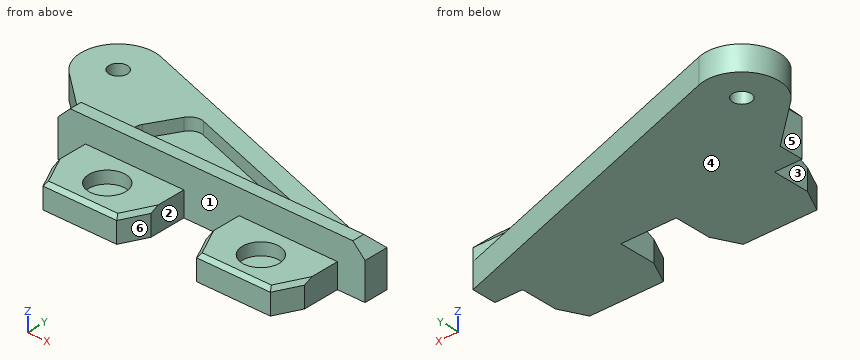
from build123d import *

# Parameters (mm, degrees)
SKIZZE1_R                       = 0.75
AUFSATZ_LINEAR_AUSTRAGEN1_DEPTH = 2
SKIZZE2_R                       = 1.5
SCHNITT_LINEAR_AUSTRAGEN1_DEPTH = 1
SKIZZE3_W                       = 25
SKIZZE3_H                       = 2
AUFSATZ_LINEAR_AUSTRAGEN2_DEPTH = 2
FASE1_SIZE                      = 1
SCHNITT_LINEAR_AUSTRAGEN2_DEPTH = 1
VERRUNDUNG1_R                   = 1
VERRUNDUNG2_R                   = 0.5
FASE2_SIZE                      = 0.3


with BuildPart() as part:
    # Skizze1 → Aufsatz-Linear austragen1 (new body)
    with BuildSketch(Plane.XY):
        with BuildLine():
            Line((9.25, -5), (3.25, -5))
            Line((3.25, -5), (2.25, -3))
            Line((2.25, -3), (2.25, 0))
            Line((2.25, 0), (0, 0))
            Line((0, 0), (0, 2))
            Line((0, 2), (-3.97861477, 5.490953701))
            ThreePointArc((-3.97861477, 5.490953701), (-4.604364731, 9.235021543), (-1.060351102, 10.595012138))
            Line((-1.060351102, 10.595012138), (25, 2))
            Line((25, 2), (25, 0))
            Line((25, 0), (22.75, 0))
            Line((22.75, 0), (22.75, -3))
            Line((22.75, -3), (21.75, -5))
            Line((21.75, -5), (15.75, -5))
            Line((15.75, -5), (14.75, -3))
            Line((14.75, -3), (14.75, 0))
            Line((14.75, 0), (10.25, 0))
            Line((10.25, 0), (10.25, -3))
            Line((10.25, -3), (9.25, -5))
        make_face()
        with Locations((-2, 7.745966692)):
            Circle(SKIZZE1_R, mode=Mode.SUBTRACT)
    extrude(amount=AUFSATZ_LINEAR_AUSTRAGEN1_DEPTH)

    # Skizze2 → Schnitt-Linear austragen1 (cut)
    with BuildSketch(Plane.XY.offset(2)):
        with Locations((6.25, -2.5)):
            Circle(SKIZZE2_R)
        with Locations(Location((18.75, -2.5, 0), (0, 0, 180))):
            Circle(SKIZZE2_R)
    extrude(amount=-SCHNITT_LINEAR_AUSTRAGEN1_DEPTH, mode=Mode.SUBTRACT)

    # Skizze3 → Aufsatz-Linear austragen2 (add)
    with BuildSketch(Plane.XY.offset(2)):
        with Locations((12.5, 1)):
            Rectangle(SKIZZE3_W, SKIZZE3_H)
    extrude(amount=AUFSATZ_LINEAR_AUSTRAGEN2_DEPTH)

    # Fase1
    fase1_edges = [part.edges().sort_by_distance(p)[0] for p in [
        (0, 1, 4),
        (25, 1, 4),
        (12.5, 2, 4),
    ]]
    chamfer(fase1_edges, length=FASE1_SIZE)

    # Skizze4 → Schnitt-Linear austragen2 (cut)
    with BuildSketch(Plane.XY.offset(2)):
        Polygon((5.059080896, 6.997274675), (18.694961237, 2.5), (2.462578152, 2.5), align=None)
    extrude(amount=-SCHNITT_LINEAR_AUSTRAGEN2_DEPTH, mode=Mode.SUBTRACT)

    # Verrundung1
    verrundung1_edges = [part.edges().sort_by_distance(p)[0] for p in [
        (2.462578152, 2.5, 1.5),
        (5.059080896, 6.997274675, 1.5),
    ]]
    fillet(verrundung1_edges, radius=VERRUNDUNG1_R)

    # Verrundung2
    verrundung2_edges = [part.edges().sort_by_distance(p)[0] for p in [
        (18.694961237, 2.5, 1.5),
    ]]
    fillet(verrundung2_edges, radius=VERRUNDUNG2_R)

    # Fase2
    fase2_edges = [part.edges().sort_by_distance(p)[0] for p in [
        (2.75, -4, 2),
        (6.25, -5, 2),
        (9.75, -4, 2),
        (15.25, -4, 2),
        (18.75, -5, 2),
        (22.25, -4, 2),
    ]]
    chamfer(fase2_edges, length=FASE2_SIZE)


solid = part.part
Geometry check sheet. Reference: the model listing, model coordinates, mm. Face numbers are marked on the shaded views. A direction names the side the tool comes from. Round coordinates to 2 decimals unless told otherwise and drop trailing zeros. Loops run counter-clockwise (first coordinate to the right, second up) from the corner with the lowest first, then second, coordinate; pieces in that order, holes last.
Item 1: Cross-section at C-C on z = 3.65. Record the boundary of the cut face in (x, y).
Item 2: Cross-section at B-B on x = -2. Record the boundary of the cut face in (y, z).
Item 3: Cross-section at D-D on x = 9.75. Record the boundary of the cut face in (y, z), then the cut area to 3 significant figures.
Item 4: Cross-section at A-A on y = -0.5. Record the boundary of the cut face in (x, z).
Item 5: Gauge pin test, flat ends, axial feed: pin 1 (1 mm diameter, centred on y = 1, z = 1, fed in from -X); pin 2 (2 mm diameter, centred on y = -1.5, z = 1, fed in from +X); pin 3 (1.5 mm diameter, centred on y = 6.5, z = 2.5, fed in from -X). Record the tip position at first contact, or that the pin passes through.
Item 6: Access from +Z, -Z, +X, -X, +Y, -Y to the whole of each face (thin tool, end or side, straight path). Record for the marked faces 1, 2 and 3.
Item 7: Thickness scan on line 1 (Y direction, x = 6.25, z = 1.35); line 2 (Y direction, x = 6.25, z = 1.75); line 3 (Z direction, x = 7.5, y = 4.25). Record the ranges inside material, lowest first.
Item 8: Mould release check, pull along X, two halves, no side actions. Record for the marked faces 4, 5 and 6: pulls with the +X half, pulls with the -X half, needs draft (parallel to the pull), parting line crosses it, or undercut.
Answer sheet:
1. outline: (0.65, 0) - (24.35, 0) - (24.35, 1.35) - (0.65, 1.35) - close
2. outline: (3.75, 0) - (7, 0) - (7, 2) - (3.75, 2) - close; (8.5, 0) - (10.75, 0) - (10.75, 2) - (8.5, 2) - close
3. outline: (-4, 0) - (7.03, 0) - (7.03, 2) - (5.45, 2) - (5.45, 1) - (2.5, 1) - (2.5, 2) - (2, 2) - (2, 3) - (1, 4) - (0, 4) - (0, 2) - (-3.33, 2) - (-4, 1.7) - close
3. area: 22.5 mm2
4. outline: (2.25, 0) - (10.25, 0) - (10.25, 2) - (2.25, 2) - close; (14.75, 0) - (22.75, 0) - (22.75, 2) - (14.75, 2) - close
5. pin 1: stops at x = 0
5. pin 2: stops at x = 22.75
5. pin 3: stops at x = -4.92
6. face 1: +Z, -Y
6. face 2: +Z, -Z, -Y
6. face 3: +Z, -Z, -X, -Y
7. line 1: y = -5 to -4, -1 to 2.5, 6.6 to 8.18
7. line 2: y = -4.95 to -4, -1 to 2.5, 6.6 to 8.18
7. line 3: z = 0 to 1
8. face 4: needs draft
8. face 5: pulls with the -X half
8. face 6: undercut
